For this review, take the finished solid that the model builds, in its own axes (mm). Give positions to 0.01 mm unless a question says otherwise; leave off trailing zeros. Order: outer loops, then holes, each group sorted by start corner. A loop starts at its lowest first (then second) coordinate and runs counter-clockwise, first axis right, second up. Notation, with made-up numbers: (18.25, 25) - (41.25, 25) arc R18 cw to (41.25, 34) - close; hole circle Ø2 at (73, 18.25). An arc over 180 degrees is marked (long way). One line per item, written item: value.
Autodesk Inventor part; units mm, degrees
ref_plane "YZ Plane" through (0, 0, 0) normal (1, 0, 0) x (0, 1, 0)
ref_plane "XZ Plane" through (0, 0, 0) normal (0, 1, 0) x (-1, 0, 0)
ref_plane "XY Plane" through (0, 0, 0) normal (0, 0, 1) x (1, 0, 0)
sketch "Эскиз1" plane through (0, 0, 0) normal (0, 1, 0) x (-1, 0, 0)
  circle A0 centre (0, 0) radius 1
  dimension "d0" = 2
sketch "Эскиз2" plane through (0, 0, 0) normal (0, 0, 1) x (1, 0, 0)
  line L0 (0, 0) -> (0, 5)
  line L1 (4, 9) -> (14, 9)
  line L2 (18, 5) -> (18, -5)
  line L3 (14, -9) -> (4, -9)
  line L4 (0, -5) -> (0, 0)
  arc A0 (4, 9) -> (0, 5) centre (4, 5) ccw
  arc A1 (18, 5) -> (14, 9) centre (14, 5) ccw
  arc A2 (14, -9) -> (18, -5) centre (14, -5) ccw
  arc A3 (0, -5) -> (4, -9) centre (4, -5) ccw
  point P0 (0, 9)
  point P1 (18, 9)
  point P2 (18, -9)
  point P3 (0, -9)
  dimension "d1" = 9
  dimension "d2" = 18
  dimension "d3" = 18
  dimension "d4" = 18
  dimension "d5" = 4
sweep "Сдвиг1" add profiles "Эскиз1" path "Эскиз2"
(1) Wall thickness on line 1 (Y direction, x = 8.75, z = -0.1); line 2 (X direction, y = 2, z = 0); line 3 (X direction, y = 3.5, z = -0.8): over which ranges is each line inside the solid? List them lowest first. Write a range as from..to.
Answers below:
line 1: y = -9.99..-8.01, 8.01..9.99
line 2: x = -1..1, 17..19
line 3: x = -0.6..0.6, 17.4..18.6
(2) Take a section at C-C (y = -2). Write out the cut boundary in (x, z).
Answers below:
outline: circle Ø2 at (0, 0); circle Ø2 at (18, 0)
(3) Take a section at B-B (x = 10.5). Write out the cut boundary in (y, z).
Answers below:
outline: circle Ø2 at (-9, 0); circle Ø2 at (9, 0)
(4) Take a section at A-A (z = 0). Write out the cut boundary in (x, y), then the cut area to 3 significant figures.
Answers below:
outline: (-1, -5) arc R5 ccw to (4, -10) - (14, -10) arc R5 ccw to (19, -5) - (19, 5) arc R5 ccw to (14, 10) - (4, 10) arc R5 ccw to (-1, 5) - close; hole (1, -5) arc R3 ccw to (4, -8) - (14, -8) arc R3 ccw to (17, -5) - (17, 5) arc R3 ccw to (14, 8) - (4, 8) arc R3 ccw to (1, 5) - close
area: 130 mm^2
(5) Draft analysis for pull direction Y (two halves, no side actions). For faces 1 (the face through (0, 0, -1)), 2 (the face through (9.1, 8.2, -0.6)), state which applies: pulls with the +Y half, pulls with the -Y half, needs draft (parallel to the pull), parting line crosses it, or undercut.
Answers below:
face 1: undercut
face 2: undercut
